Verification items for the finished model (mm, model axes). A direction names the side the tool comes from. Coordinates: 2 decimals unless noted, no trailing zeros. Order: outer loops, then holes, each group sorted by start corner. A loop starts at its lowest first (then second) coordinate and runs counter-clockwise, first axis right, second up. Notation, with made-up numbers: (61, 22.25) -> (98, 22.25) arc R10 cw to (98, 29.25) -> close; hole circle Ø4 at (20, 12.25). An arc over 180 degrees is marked (long way). Answer as CSV lines item,"result".
```python
from build123d import *

# Parameters (mm, degrees)
SKETCH1_W           = 12.446
SKETCH1_H           = 22.098
BOSS_EXTRUDE1_DEPTH = 22.86
SKETCH2_W           = 12.446
SKETCH2_H           = 2.032
BOSS_EXTRUDE2_DEPTH = 2.032
CUT_EXTRUDE1_DEPTH  = 2.032
BOSS_EXTRUDE3_DEPTH = 8.89
SKETCH5_R           = 2.54
CUT_EXTRUDE2_DEPTH  = 1.27


with BuildPart() as part:
    # Sketch1 → Boss-Extrude1 (new body)
    with BuildSketch(Plane.XY):
        Rectangle(SKETCH1_W, SKETCH1_H)
    extrude(amount=BOSS_EXTRUDE1_DEPTH)

    # Sketch2 → Boss-Extrude2 (add)
    with BuildSketch(Plane(origin=(0, 11.049, 0), x_dir=(1, 0, 0), z_dir=(0, 1, 0))):
        with Locations((0, -2.032)):
            Rectangle(SKETCH2_W, SKETCH2_H)
    boss_extrude2 = extrude(amount=BOSS_EXTRUDE2_DEPTH)

    # Sketch3 → Cut-Extrude1 (cut)
    with BuildSketch(Plane(origin=(0, 0, 1.016), x_dir=(-1, 0, 0), z_dir=(0, 0, -1))):
        with BuildLine():
            Line((-0.381, 13.081), (-0.381, 12.507864133))
            ThreePointArc((-0.381, 12.507864133), (0, 11.4808), (0.381, 12.507864133))
            Line((0.381, 12.507864133), (0.381, 13.081))
            Line((0.381, 13.081), (-0.381, 13.081))
        make_face()
    cut_extrude1 = extrude(amount=-CUT_EXTRUDE1_DEPTH, mode=Mode.SUBTRACT)

    # Mirror1: Boss-Extrude2 across plane
    add(boss_extrude2.mirror(Plane.ZX))

    # Mirror2: Cut-Extrude1 across plane
    add(cut_extrude1.mirror(Plane.ZX), mode=Mode.SUBTRACT)

    # Sketch4 → Boss-Extrude3 (add)
    with BuildSketch(Plane(origin=(0, 0, 0), x_dir=(-1, 0, 0), z_dir=(0, 0, -1))):
        with BuildLine():
            ThreePointArc((-2.967141975, 0.644082038), (0, -11.049), (2.967141975, 0.644082038))
            ThreePointArc((2.967141975, 0.644082038), (0, 4.389486154), (-2.967141975, 0.644082038))
        make_face()
    extrude(amount=BOSS_EXTRUDE3_DEPTH)

    # Sketch5 → Cut-Extrude2 (cut)
    with BuildSketch(Plane(origin=(0, 0, -8.89), x_dir=(-1, 0, 0), z_dir=(0, 0, -1))):
        with Locations((0, -4.826)):
            Circle(SKETCH5_R)
    extrude(amount=-CUT_EXTRUDE2_DEPTH, mode=Mode.SUBTRACT)


solid = part.part
```
Item 1: Thickness scan on line 1 (Y direction, x = -4.25, z = 5); line 2 (Y direction, x = 0, z = 1.7); line 3 (Y direction, x = 0, z = -8.2). Record the ranges inside material, lowest first.
Answer list:
line 1,"-11.05 to 11.05"
line 2,"-11.48 to 11.48"
line 3,"-11.05 to -7.37, -2.29 to 4.39"
Item 2: Section check D-D, the plane x = 5.25. Record the boundary of the cut face in (y, z), plus the area to 3 significant figures.
Answer list:
outline,"(-13.08, 1.02) -> (-11.05, 1.02) -> (-11.05, 0) -> (-8.17, 0) -> (-8.17, -8.89) -> (-1.48, -8.89) -> (-1.48, 0) -> (11.05, 0) -> (11.05, 1.02) -> (13.08, 1.02) -> (13.08, 3.05) -> (11.05, 3.05) -> (11.05, 22.86) -> (-11.05, 22.86) -> (-11.05, 3.05) -> (-13.08, 3.05) -> close"
area,"573 mm2"
Item 3: Release check for a two-part mould opening along X. For faces 5 (the flat face through (3, -13.081, 2)), 6 (the flat face through (6.223, 0, 11)), 7 (the flat face through (0, -5, -7.62)) record: +X half, -X half, draft (parallel to the pull), parting line (faces both ways), or undercut.
Answer list:
face 5,"draft"
face 6,"+X half"
face 7,"undercut"
Item 4: Section check A-A, the plane y = -8.25. Record the boundary of the cut face in (x, z).
Answer list:
outline,"(-6.22, 0) -> (-5.2, 0) -> (-5.2, -8.89) -> (5.2, -8.89) -> (5.2, 0) -> (6.22, 0) -> (6.22, 22.86) -> (-6.22, 22.86) -> close"
Item 5: Tool access check on faces 1 (the flat face through (-1, 12, 3.048)), 2 (the flat face through (-0.1, 11.049, 0.5)), 3 (the flat face through (0, 7, 0)), 4 (the flat face through (-1, -12, 1.016)). Record the directions out of +Z, -Z, +X, -X, +Y, -Y that give a thin tool (end or side, any length) a straight path to the whole face; none if there is none.
Answer list:
face 1,"+Z, +X, -X, +Y"
face 2,"-Z, +X, -X, +Y"
face 3,"-Z, +Y"
face 4,"-Z, +X, -X, -Y"
Item 6: Section check B-B, the plane x = -4. Record the boundary of the cut face in (y, z), plus the area to 3 significant figures.
Answer list:
outline,"(-13.08, 1.02) -> (-11.05, 1.02) -> (-11.05, 0) -> (-9.59, 0) -> (-9.59, -8.89) -> (-0.06, -8.89) -> (-0.06, 0) -> (11.05, 0) -> (11.05, 1.02) -> (13.08, 1.02) -> (13.08, 3.05) -> (11.05, 3.05) -> (11.05, 22.86) -> (-11.05, 22.86) -> (-11.05, 3.05) -> (-13.08, 3.05) -> close"
area,"598 mm2"
Item 7: Section check C-C, the plane z = 11.5. Record the boundary of the cut face in (x, y).
Answer list:
outline,"(-6.22, -11.05) -> (6.22, -11.05) -> (6.22, 11.05) -> (-6.22, 11.05) -> close"
Item 8: Depth check by flat-ended pin: pin 1 Ø1.5 at (x, y) = (0, -12.065) entering from -Z; pin 2 Ø1.5 at (x, y) = (0, -6) entering from -Z; pin 3 Ø6 at (x, z) = (-1.5, 9.5) entering from +Y. Enter the tip coordinate at first touch or a pass-through.
Answer list:
pin 1,"z = 1.02"
pin 2,"z = -7.62"
pin 3,"y = 11.05"
